The listing builds one solid part. Answer for the finished solid, in the listing's coordinates (mm). Face numbers are marked on the shaded views. A direction names the side the tool comes from. Round coordinates to 2 decimals unless told otherwise and drop trailing zeros. Write each loop counter-clockwise with the first axis right and the second up, starting at its lowest first coordinate (ties: lowest second). Pieces come first, ordered by that corner, then holes.
Item 1: A tool of negligible diameter and unlimited length cuts with its end or side. For the marked faces 1, 2, 3 and 4, from which of +Z, -Z, +X, -X, +Y, -Y can it reach the whole face along a straight path? Write none if from no direction.
Item 2: Find section A-A on z = -2.5. Give the vertices of the cut face in (x, y).
Item 3: Find the intervals of material crossed by probe 1 along Y at (x, z) = (1.5, -3.25); probe 2 along Z at (x, y) = (-5.5, 3.75); probe 3 along X at (y, z) = (1, -2), in increasing order.
Item 4: Each of these flat-tipped pins is pushed along its axis until it touches: pin 1 (0.8 mm diameter, centred on y = 1.5, z = 3.5, fed in from +X); pin 2 (1.1 mm diameter, centred on x = 0, z = 3, fed in from -Y); pin 3 (4 mm diameter, centred on y = 4, z = 1, fed in from +X). Where does it stop, or does it pass through?
Item 5: Find section C-C on x = 0. Give the vertices of the cut face in (y, z), then the cut area to 3 significant figures.
Item 6: Find section B-B on y = 0. Give the vertices of the cut face in (x, z), then the cut area to 3 significant figures.
Item 7: Find section D-D on z = 1.5. Give the vertices of the cut face in (x, y), then the cut area to 3 significant figures.
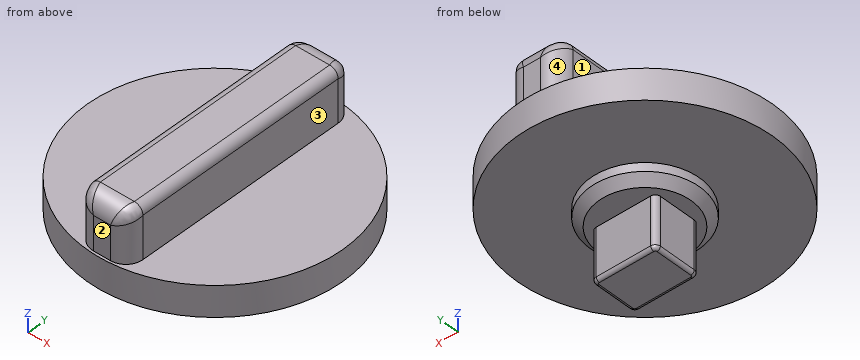
```python
from build123d import *

# Parameters (mm, degrees)
SKETCH008_R     = 7.5
PAD004_DEPTH    = 1.8
SKETCH009_W     = 3
SKETCH009_H     = 14.696938
PAD005_DEPTH    = 3
SKETCH010_R     = 3.2
PAD006_DEPTH    = 1
CHAMFER003_SIZE = 0.5
SKETCH011_W     = 3.8
SKETCH011_H     = 2.8
PAD007_DEPTH    = 3
FILLET004_R     = 0.3
FILLET005_R     = 0.2
FILLET006_R     = 0.5
FILLET_R        = 1
FILLET007_R     = 1


with BuildPart() as part:
    # Sketch008 → Pad004 (new body)
    with BuildSketch(Plane.XY):
        Circle(SKETCH008_R)
    extrude(amount=PAD004_DEPTH)

    # Sketch009 (on Face3 of Pad004) → Pad005 (join)
    with BuildSketch(Plane.XY.offset(1.8)):
        Rectangle(SKETCH009_W, SKETCH009_H)
    extrude(amount=PAD005_DEPTH)

    # Sketch010 → Pad006 (join)
    with BuildSketch(Plane(origin=(0, 0, 0), x_dir=(1, 0, 0), z_dir=(0, 0, -1))):
        Circle(SKETCH010_R)
    extrude(amount=PAD006_DEPTH)

    # Chamfer003
    chamfer003_edges = [part.edges().sort_by_distance(p)[0] for p in [
        (-3.2, 0, -1),
    ]]
    chamfer(chamfer003_edges, length=CHAMFER003_SIZE)

    # Sketch011 (on Face4 of Chamfer003) → Pad007 (join)
    with BuildSketch(Plane(origin=(0, 0, -1), x_dir=(1, 0, 0), z_dir=(0, 0, -1))):
        Rectangle(SKETCH011_W, SKETCH011_H)
    extrude(amount=PAD007_DEPTH)

    # Fillet004
    fillet004_edges = [part.edges().sort_by_distance(p)[0] for p in [
        (-1.9, 1.4, -2.5),
        (-1.9, -1.4, -2.5),
        (1.9, 1.4, -2.5),
        (1.9, -1.4, -2.5),
    ]]
    fillet(fillet004_edges, radius=FILLET004_R)

    # Fillet005
    fillet005_edges = [part.edges().sort_by_distance(p)[0] for p in [
        (0, -1.4, -4),
        (1.812132, -1.312132, -4),
        (1.9, 0, -4),
        (1.812132, 1.312132, -4),
        (0, 1.4, -4),
        (-1.812132, 1.312132, -4),
        (-1.9, 0, -4),
        (-1.812132, -1.312132, -4),
    ]]
    fillet(fillet005_edges, radius=FILLET005_R)

    # Fillet006
    fillet006_edges = [part.edges().sort_by_distance(p)[0] for p in [
        (-1.5, 0, 4.8),
        (1.5, 0, 4.8),
    ]]
    fillet(fillet006_edges, radius=FILLET006_R)

    # Fillet
    fillet_edges = [part.edges().sort_by_distance(p)[0] for p in [
        (-1.5, -7.348469, 3.05),
        (1.5, -7.348469, 3.05),
        (1.353553, -7.348469, 4.653553),
        (0, -7.348469, 4.8),
        (-1.353553, -7.348469, 4.653553),
    ]]
    fillet(fillet_edges, radius=FILLET_R)

    # Fillet007
    fillet007_edges = [part.edges().sort_by_distance(p)[0] for p in [
        (1.5, 7.348469, 3.05),
        (1.353553, 7.348469, 4.653553),
        (0, 7.348469, 4.8),
        (-1.353553, 7.348469, 4.653553),
        (-1.5, 7.348469, 3.05),
    ]]
    fillet(fillet007_edges, radius=FILLET007_R)


solid = part.part
```
Check values:
1. face 1: +Z, -X, +Y, -Y
1. face 2: +Z, +X, -X, -Y
1. face 3: +Z, +X, +Y, -Y
1. face 4: +Z, -X, +Y
2. outline: (-1.9, -1.1) arc R0.3 ccw to (-1.6, -1.4) - (1.6, -1.4) arc R0.3 ccw to (1.9, -1.1) - (1.9, 1.1) arc R0.3 ccw to (1.6, 1.4) - (-1.6, 1.4) arc R0.3 ccw to (-1.9, 1.1) - close
3. probe 1: y = -1.4 to 1.4
3. probe 2: z = 0 to 1.8
3. probe 3: x = -1.9 to 1.9
4. pin 1: stops at x = 1.5
4. pin 2: stops at y = -7.35
4. pin 3: stops at x = 7.23
5. outline: (-7.5, 0) - (-3.2, 0) - (-3.2, -0.5) - (-2.7, -1) - (-1.4, -1) - (-1.4, -3.8) arc R0.2 ccw to (-1.2, -4) - (1.2, -4) arc R0.2 ccw to (1.4, -3.8) - (1.4, -1) - (2.7, -1) - (3.2, -0.5) - (3.2, 0) - (7.5, 0) - (7.5, 1.8) - (7.35, 1.8) - (7.35, 3.8) arc R1 ccw to (6.35, 4.8) - (-6.35, 4.8) arc R1 ccw to (-7.35, 3.8) - (-7.35, 1.8) - (-7.5, 1.8) - close
5. area: 85.2 mm2
6. outline: (-7.5, 0) - (-3.2, 0) - (-3.2, -0.5) - (-2.7, -1) - (-1.9, -1) - (-1.9, -3.8) arc R0.2 ccw to (-1.7, -4) - (1.7, -4) arc R0.2 ccw to (1.9, -3.8) - (1.9, -1) - (2.7, -1) - (3.2, -0.5) - (3.2, 0) - (7.5, 0) - (7.5, 1.8) - (1.5, 1.8) - (1.5, 4.3) arc R0.5 ccw to (1, 4.8) - (-1, 4.8) arc R0.5 ccw to (-1.5, 4.3) - (-1.5, 1.8) - (-7.5, 1.8) - close
6. area: 53.4 mm2
7. outline: circle Ø15 at (0, 0)
7. area: 177 mm2
